The figure shows three views and two pictorial views of one solid part (mm, origin at its lowest corner). Answer the questions. Round coordinates to 2 decimals unless told otherwise and drop trailing zeros. Order: outer loops, then holes, each group sorted by start corner. A loop starts at its lowest first (then second) coordinate and runs counter-clockwise, first axis right, second up. Notation, with made-up numbers: (40, 47.25) - (75, 47.25) arc R24 ccw to (75, 79.25) - close; hole circle Ø11 at (82, 22.25). An arc over 180 degrees is marked (long way). Answer in a Markdown table with one row per item.
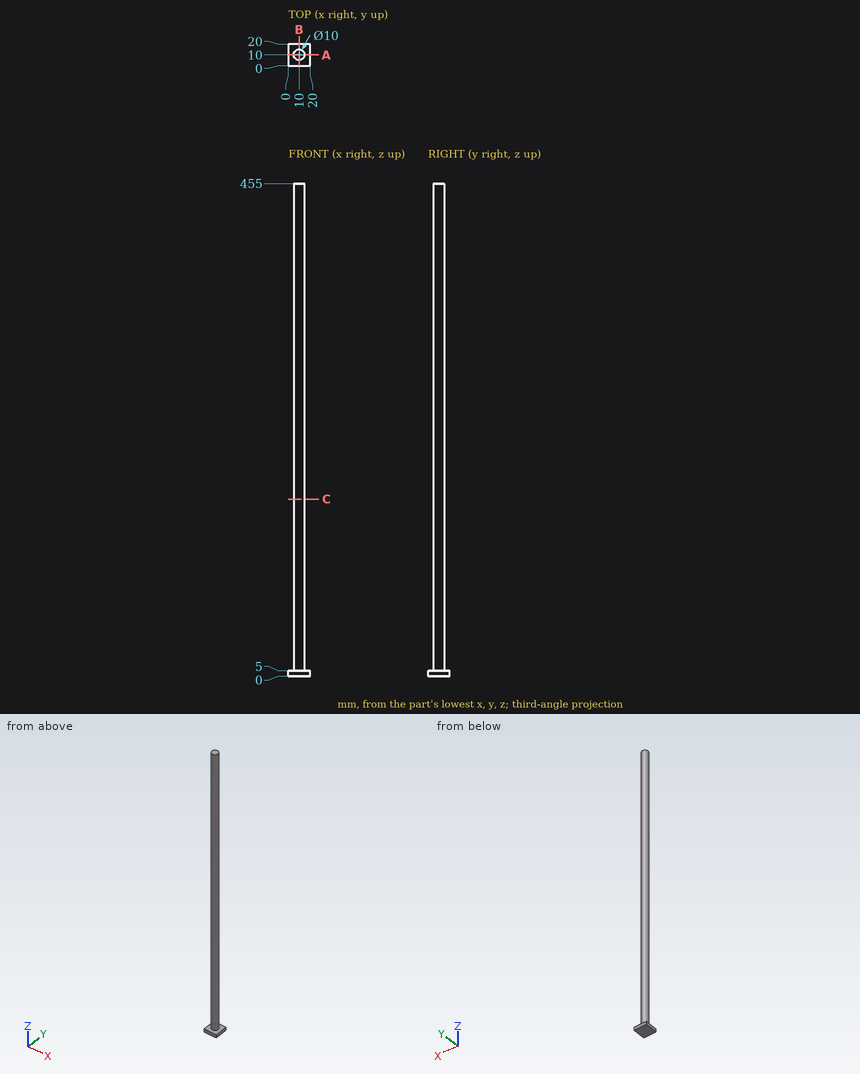
1) Find the intervals of material crossed by probe 1 along Z at (x, y) = (13, 3.25); probe 2 along Y at (x, z) = (10, 132); probe 3 along X at (y, z) = (10.75, 269.5), in increasing order. Write a range as from..to.
Filled in:
| item | result |
|---|---|
| probe 1 | z = 0..5 |
| probe 2 | y = 5..15 |
| probe 3 | x = 5.06..14.94 |
2) Each of these flat-tipped pins is pushed along its axis until it touches: pin 1 (2 mm diameter, centred on x = 6.5, z = 207.5, fed in from +Y); pin 2 (10 mm diameter, centred on y = 6.5, z = 184, fed in from -X); pin 3 (10 mm diameter, centred on x = 9.5, z = 377.5, fed in from +Y); pin 4 (6 mm diameter, centred on x = 4.5, y = 14.5, fed in from -Z). Where does it stop, or does it pass through?
Filled in:
| item | result |
|---|---|
| pin 1 | stops at y = 14.33 |
| pin 2 | stops at x = 5 |
| pin 3 | stops at y = 15 |
| pin 4 | stops at z = 0 |
3) Find section C-C, the plane z = 163.5. Give the vertices of the cut face in (x, y), then the cut area to 3 significant figures.
Filled in:
| item | result |
|---|---|
| outline | circle Ø10 at (10, 10) |
| area | 78.5 mm^2 |
4) Find section A-A, the plane y = 10. Give the vertices of the cut face in (x, z), then the cut area to 3 significant figures.
Filled in:
| item | result |
|---|---|
| outline | (0, 0) - (20, 0) - (20, 5) - (15, 5) - (15, 455) - (5, 455) - (5, 5) - (0, 5) - close |
| area | 4,600 mm^2 |
